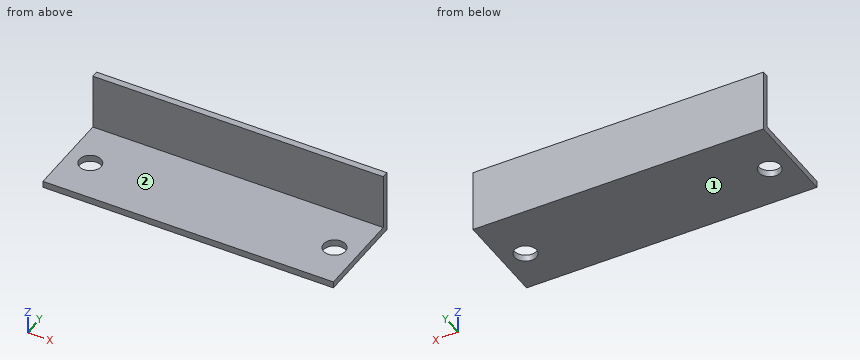
```python
from build123d import *

# Parameters (mm, degrees)
F0_W     = 44
F0_H     = 14.4
F1_DEPTH = 9.5
F2_W     = 13.4
F2_H     = 8.5
F3_DEPTH = 44
F5_D     = 3.3


with BuildPart() as f1:
    # F0 (on Top) → F1 (new body)
    with BuildSketch(Plane.XY):
        with Locations((1.3719686568, -36.0766266167)):
            Rectangle(F0_W, F0_H)
    extrude(amount=F1_DEPTH)

    # F2 (on face) → F3 (cut)
    with BuildSketch(Plane.YZ.offset(23.3719686568)):
        with Locations((-36.5766266167, 5.25)):
            Rectangle(F2_W, F2_H)
    extrude(amount=-F3_DEPTH, mode=Mode.SUBTRACT)

    # F5 (through all)
    with Locations(Plane.XY.offset(1)):
        with Locations((-17.1280313432, -36.7766266167), (19.8719686568, -36.7766266167)):
            Hole(F5_D / 2)


solid = f1.part
```
Here's how the part is built. I have some questions about the finished solid (model axes, mm). Face numbers are marked on the shaded views. A direction names the side the tool comes from. Coordinates: 2 decimals unless noted, no trailing zeros. Write each loop counter-clockwise with the first axis right and the second up, starting at its lowest first coordinate (ties: lowest second). Pieces come first, ordered by that corner, then holes. Notation, with made-up numbers: (-39, -34) - (-22, -34) arc R31 ccw to (-22, -2) - close; hole circle Ø8 at (4, -28.5). An arc over 180 degrees is marked (long way). One line per item, written item: value.
1) Suppose I cut it at C-C on z = 8.5. Write out the boundary of the cut face in (x, y), and give its area (3 significant figures).
Model answer:
outline: (-20.63, -29.88) - (23.37, -29.88) - (23.37, -28.88) - (-20.63, -28.88) - close
area: 44.0 mm²
2) Suppose I cut it at A-A on y = -36.25. Write out the boundary of the cut face in (x, z), and give its area (3 significant figures).
Model answer:
outline: (-20.63, 0) - (-18.69, 0) - (-18.69, 1) - (-20.63, 1) - close; (-15.56, 0) - (18.31, 0) - (18.31, 1) - (-15.56, 1) - close; (21.44, 0) - (23.37, 0) - (23.37, 1) - (21.44, 1) - close
area: 37.7 mm²
3) I need wall thicknesses on line 1 along Y through (x, z) = (18.5, 7.5); line 2 along Z through (x, y) = (16, -42.5). Which ranges of each line are inside material? Lowest first, please.
Model answer:
line 1: y = -29.88 to -28.88
line 2: z = 0 to 1
4) I'm going to push flat-ended pins straight in: P1, Ø2.5, axis at x = -17.13, y = -36.78, coming from the -Z side (3 decimals); P2, Ø5.5, axis at x = 19.87, y = -36.78, coming from the +Z side; P3, Ø1.5, axis at x = 11, z = 8.5, coming from the -Y side. Where does each tip first touch, or does it pass through?
Model answer:
P1: passes through
P2: stops at z = 1
P3: stops at y = -29.88
5) Suppose I cut it at D-D on x = -17.5. Write out the boundary of the cut face in (y, z), and give its area (3 significant figures).
Model answer:
outline: (-43.28, 0) - (-38.38, 0) - (-38.38, 1) - (-43.28, 1) - close; (-35.17, 0) - (-28.88, 0) - (-28.88, 9.5) - (-29.88, 9.5) - (-29.88, 1) - (-35.17, 1) - close
area: 19.7 mm²
6) Suppose I cut it at B-B on x = 15.5. Write out the boundary of the cut face in (y, z).
Model answer:
outline: (-43.28, 0) - (-28.88, 0) - (-28.88, 9.5) - (-29.88, 9.5) - (-29.88, 1) - (-43.28, 1) - close
7) On a 3-axis mill with a long thin cutter (end or side, diameter ignored), from which of +Z, -Z, +X, -X, +Y, -Y can I reach the whole of each face in a straight line? I mean the marked faces 1 and 2. Say none if no direction works.
Model answer:
face 1: -Z, +X, -X, +Y, -Y
face 2: +Z, +X, -X, -Y
